Source: CAD feature listing. Evaluate the final solid. Frame: model axes, mm. A direction names the side the tool comes from. Give positions to 0.01 mm unless a question says otherwise; leave off trailing zeros. Order: outer loops, then holes, each group sorted by start corner. A loop starts at its lowest first (then second) coordinate and runs counter-clockwise, first axis right, second up. Notation, with made-up numbers: (49.25, 82) -> (87.25, 82) arc R8 cw to (87.25, 88) -> close; hole circle Ø7 at (59, 28). An arc over 180 degrees is marked (long way). Answer in a Markdown table with one row per item.
Autodesk Inventor part; units mm, degrees
ref_plane "YZ Plane" through (0, 0, 0) normal (1, 0, 0) x (0, 1, 0)
ref_plane "XZ Plane" through (0, 0, 0) normal (0, 1, 0) x (-1, 0, 0)
ref_plane "XY Plane" through (0, 0, 0) normal (0, 0, 1) x (1, 0, 0)
sketch "Sketch1" plane through (0, 0, 0) normal (0, 1, 0) x (-1, 0, 0)
  line L0 (-3, 13) -> (3, 13)
  line L1 (3, 13) -> (3, -13)
  line L2 (3, -13) -> (-3, -13)
  line L3 (-3, -13) -> (-3, 13)
  line L4 (-3, 13) -> (3, -13) construction
  line L5 (3, 13) -> (-3, -13) construction
  point P0 (0, 0)
  dimension "d0" = 6
  dimension "d1" = 26
extrude "Extrusion1" add sketch "Sketch1" along normal blind 4
sketch "Sketch2" plane through (3, 0, -13) normal (0, 0, -1) x (-1, 0, 0)
  line L0 (0, 0) -> (6, 0)
  line L1 (6, 0) -> (-12, 0)
  line L2 (-12, 0) -> (-12, 4)
  line L3 (-12, 4) -> (6, 4)
  line L4 (6, 4) -> (6, 0)
  point P0 (3, 0)
  dimension "d4" = 18
  dimension "d5" = 4
extrude "Extrusion2" add sketch "Sketch2" along normal blind 4
sketch "Sketch3" plane through (0, 4, 0) normal (0, 1, 0) x (1, 0, 0)
  line L0 (3, -13) -> (3, 13)
  line L1 (3, 13) -> (0, 13)
  line L2 (0, 13) -> (0, 8)
  line L3 (0, 8) -> (0, -2)
  circle A0 centre (0, 8) radius 1.1
  circle A1 centre (0, -2) radius 1.1
  point P0 (0, 0)
  dimension "d8" = 5
  dimension "d9" = 10
  dimension "d10" = 2.2
  dimension "d11" = 2.2
extrude "Extrusion3" cut sketch "Sketch3" against normal up to next
sketch "Sketch4" plane through (0, 4, 0) normal (0, 1, 0) x (1, 0, 0)
  line L0 (3, 13) -> (3, -13)
  line L1 (-3, -13) -> (-3, 17)
  line L2 (3, -13) -> (-3, -13)
  line L3 (-3, -13) -> (-3, -5)
  line L4 (-3, -5) -> (3, -5)
  line L5 (3, -5) -> (3, -13)
  point P0 (0, 0)
  dimension "d14" = 8
extrude "Extrusion4" cut sketch "Sketch4" against normal blind 4
fillet "Fillet1" radius 3 2 edges at (3, 2, 5) (-3, 2, 5)
sketch "Sketch5" plane through (0, 4, 0) normal (0, 1, 0) x (1, 0, 0)
  line L0 (15, 13) -> (11.1, 13)
  line L1 (3, 13) -> (15, 13)
  line L2 (11.1, 13) -> (11.1, 11.5)
  line L3 (11.1, 11.5) -> (15, 13)
  point P0 (0, 0)
  dimension "d18" = 3.9
  dimension "d19" = 1.5
extrude "Extrusion5" add sketch "Sketch5" against normal blind 4
fillet "Fillet2" radius 1 1 edges at (11.1, 2, -11.5)
fillet "Fillet3" radius 3 1 edges at (-3, 2, -17)
sketch "Sketch6" plane through (0, 4, 0) normal (0, 1, 0) x (1, 0, 0)
  line L0 (0, 17) -> (15, 17)
  line L1 (3.0924, 17) -> (4.5066, 15.5858)
  line L2 (3.0924, 17) -> (5.0924, 17) construction
  line L3 (4.5066, 15.5858) -> (5.9208, 17)
  line L4 (5.9208, 17) -> (7.335, 15.5858)
  line L5 (5.9208, 17) -> (7.9208, 17) construction
  line L6 (7.335, 15.5858) -> (8.7492, 17)
  point P0 (0, 0)
  dimension "d24" = 2
  dimension "d25" = 45
  dimension "d26" = 2
  dimension "d27" = 45
extrude "Extrusion6" cut sketch "Sketch6" against normal up to next
fillet "Fillet4" radius 1 5 edges at (3.0924, 2, -17) (4.5066, 2, -15.5858) (5.9208, 2, -17) (7.335, 2, -15.5858) (8.7492, 2, -17)
fillet "Fillet5" radius 2.5 2 edges at (15, 2, -17) (15, 2, -13)
properties part number "arm_lock" material "Nylon 6/6"
(1) First-contact query: pin 1 Ø1.2 at (y, z) = (2, -8) entering from +X. Flat tip, straight axial feed; report the tip coordinate or a pass-through.
A:
| item | result |
|---|---|
| pin 1 | stops at x = 3 |
(2) Access query for faces 5 (the flat face through (7, 2, -13)), 6 (the cylindrical face through (-2.1, 1.97, 4.14)). Directions: +Z, -Z, +X, -X, +Y, -Y. A direction counts if a zero-diameter tool reaches every point of the face in a straight line with its end or side. Return the directions, or none.
A:
| item | result |
|---|---|
| face 5 | +Z, +Y, -Y |
| face 6 | +Z, -X, +Y, -Y |
(3) Section query A-A (z = -8). Return the cut outline in (x, y).
A:
| item | result |
|---|---|
| outline | (-3, 0) -> (-1.1, 0) -> (-1.1, 4) -> (-3, 4) -> close; (1.1, 0) -> (3, 0) -> (3, 4) -> (1.1, 4) -> close |
(4) Section query B-B (y = 0.5). Give the number of separate pieces and of enclosed holes in the cut face, plus the area to 3 significant figures.
A:
| item | result |
|---|---|
| separate pieces | 1 |
| enclosed holes | 2 |
| area | 161 mm^2 |
(5) Section query C-C (z = -5.5). Return the cut outline in (x, y), plus the area to 3 significant figures.
A:
| item | result |
|---|---|
| outline | (-3, 0) -> (3, 0) -> (3, 4) -> (-3, 4) -> close |
| area | 24.0 mm^2 |
(6) Ray query, probe 1 along Z at (x, y) = (0, 2.6); probe 2 along X at (y, z) = (2.4, 2); probe 3 along Z at (x, y) = (-1, 3.2). Return the intervals inside material, ascending.
A:
| item | result |
|---|---|
| probe 1 | z = -17 to -9.1, -6.9 to 0.9, 3.1 to 5 |
| probe 2 | x = -3 to -1.1, 1.1 to 3 |
| probe 3 | z = -16.83 to -8.46, -7.54 to 1.54, 2.46 to 4.83 |
(7) Section query D-D (x = 6). Return the cut outline in (y, z).
A:
| item | result |
|---|---|
| outline | (0, -16.58) -> (4, -16.58) -> (4, -13) -> (0, -13) -> close |
(8) Pull-direction query (X, two-part tool) for faces 1 (the cylindrical face through (2.14, 1.97, 4.1)), 2 (the flat face through (-3, 2, -6)), 3 (the flat face through (2, 0, -9)), 4 (the cylindrical face through (-0.238, 2.028, -6.926)); classes: +X half, -X half, draft (parallel to the pull), parting line (faces both ways), or undercut.
A:
| item | result |
|---|---|
| face 1 | +X half |
| face 2 | -X half |
| face 3 | draft |
| face 4 | undercut |
